from build123d import *

# Parameters (mm, degrees)
CUT_EXTRUDE1_REACH      = 157
SKETCH2_R               = 6
BOSS_EXTRUDE1_DEPTH     = 633
BOSS_EXTRUDE2_DEPTH     = 5
SKETCH6_W               = 63
SKETCH6_H               = 200
BOSS_EXTRUDE3_DEPTH     = 5
BOSS_EXTRUDE4_DEPTH     = 100
CUT_EXTRUDE2_DEPTH      = 128
CUT_EXTRUDE2_DEPTH_BACK = 81


with BuildPart() as part:
    # Sketch1 → Revolve1 (revolve)
    with BuildSketch(Plane(origin=(0, 0, 0), x_dir=(1, 0, 0), z_dir=(0, 1, 0))):
        Polygon((825, 0), (825, 80), (813, 80), (813, 52.102452079), (763.258124913, 43.215384463), (763.258124913, 48.450903374), (746.851230852, 48.450903374), (746.851230852, 33.013608417), (670, 33.013608417), (670, 0), align=None)
    revolve(axis=Axis((657.896171738, 0, 0), (1, 0, 0)))

    # Sketch2 → Cut-Extrude1 (cut, up to next)
    with BuildSketch(Plane(origin=(825, 0, 0), x_dir=(0, 0, -1), z_dir=(1, 0, 0)), mode=Mode.PRIVATE) as cut_extrude1_sk1:
        with Locations((0, 66)):
            Circle(SKETCH2_R)
    cut_extrude1_tool1 = extrude(cut_extrude1_sk1.sketch, amount=-CUT_EXTRUDE1_REACH, mode=Mode.PRIVATE) & part.part
    add(cut_extrude1_tool1.solids().sort_by_distance((825, 66, 0))[0], mode=Mode.SUBTRACT)
    # Sketch2 → Cut-Extrude1 (cut, up to next)
    with BuildSketch(Plane(origin=(825, 0, 0), x_dir=(0, 0, -1), z_dir=(1, 0, 0)), mode=Mode.PRIVATE) as cut_extrude1_sk2:
        with Locations((62.769730075, 20.395121629)):
            Circle(SKETCH2_R)
    cut_extrude1_tool2 = extrude(cut_extrude1_sk2.sketch, amount=-CUT_EXTRUDE1_REACH, mode=Mode.PRIVATE) & part.part
    add(cut_extrude1_tool2.solids().sort_by_distance((825, 20.395122, -62.76973))[0], mode=Mode.SUBTRACT)
    # Sketch2 → Cut-Extrude1 (cut, up to next)
    with BuildSketch(Plane(origin=(825, 0, 0), x_dir=(0, 0, -1), z_dir=(1, 0, 0)), mode=Mode.PRIVATE) as cut_extrude1_sk3:
        with Locations((38.793826651, -53.395121629)):
            Circle(SKETCH2_R)
    cut_extrude1_tool3 = extrude(cut_extrude1_sk3.sketch, amount=-CUT_EXTRUDE1_REACH, mode=Mode.PRIVATE) & part.part
    add(cut_extrude1_tool3.solids().sort_by_distance((825, -53.395122, -38.793827))[0], mode=Mode.SUBTRACT)
    # Sketch2 → Cut-Extrude1 (cut, up to next)
    with BuildSketch(Plane(origin=(825, 0, 0), x_dir=(0, 0, -1), z_dir=(1, 0, 0)), mode=Mode.PRIVATE) as cut_extrude1_sk4:
        with Locations((-38.793826651, -53.395121629)):
            Circle(SKETCH2_R)
    cut_extrude1_tool4 = extrude(cut_extrude1_sk4.sketch, amount=-CUT_EXTRUDE1_REACH, mode=Mode.PRIVATE) & part.part
    add(cut_extrude1_tool4.solids().sort_by_distance((825, -53.395122, 38.793827))[0], mode=Mode.SUBTRACT)
    # Sketch2 → Cut-Extrude1 (cut, up to next)
    with BuildSketch(Plane(origin=(825, 0, 0), x_dir=(0, 0, -1), z_dir=(1, 0, 0)), mode=Mode.PRIVATE) as cut_extrude1_sk5:
        with Locations((-62.769730075, 20.395121629)):
            Circle(SKETCH2_R)
    cut_extrude1_tool5 = extrude(cut_extrude1_sk5.sketch, amount=-CUT_EXTRUDE1_REACH, mode=Mode.PRIVATE) & part.part
    add(cut_extrude1_tool5.solids().sort_by_distance((825, 20.395122, 62.76973))[0], mode=Mode.SUBTRACT)


with BuildPart() as body_2:
    # Sketch4 → Boss-Extrude1 (new body)
    with BuildSketch(Plane(origin=(0, 0, 0), x_dir=(0, 0, -1), z_dir=(1, 0, 0))):
        with BuildLine():
            Line((-185, 107), (-105, 107))
            ThreePointArc((-105, 107), (-97.928932188, 104.071067812), (-95, 97))
            Line((-95, 97), (-95, 37))
            ThreePointArc((-95, 37), (-97.928932188, 29.928932188), (-105, 27))
            Line((-105, 27), (-185, 27))
            ThreePointArc((-185, 27), (-192.071067812, 29.928932188), (-195, 37))
            Line((-195, 37), (-195, 97))
            ThreePointArc((-195, 97), (-192.071067812, 104.071067812), (-185, 107))
        make_face()
    extrude(amount=BOSS_EXTRUDE1_DEPTH)

    # Sketch5 → Boss-Extrude2 (add)
    with BuildSketch(Plane(origin=(633, 0, 0), x_dir=(0, 0, -1), z_dir=(1, 0, 0))):
        Polygon((-245, 127), (-45, 127), (-45, 67), (-115, -3), (-175, -3), (-245, 67), align=None)
    extrude(amount=-BOSS_EXTRUDE2_DEPTH)

    # Sketch6 → Boss-Extrude3 (add)
    with BuildSketch(Plane(origin=(0, 127, 0), x_dir=(1, 0, 0), z_dir=(0, 1, 0))):
        with Locations((601.5, -145)):
            Rectangle(SKETCH6_W, SKETCH6_H)
        with BuildLine():
            Line((595, -58), (605, -58))
            ThreePointArc((605, -58), (612, -65), (605, -72))
            Line((605, -72), (595, -72))
            ThreePointArc((595, -72), (588, -65), (595, -58))
        make_face(mode=Mode.SUBTRACT)
        with BuildLine():
            Line((595, -232), (605, -232))
            ThreePointArc((605, -232), (612, -225), (605, -218))
            Line((605, -218), (595, -218))
            ThreePointArc((595, -218), (588, -225), (595, -232))
        make_face(mode=Mode.SUBTRACT)
    extrude(amount=-BOSS_EXTRUDE3_DEPTH)


with BuildPart() as body_3:
    # Sketch7 → Boss-Extrude4 (new body)
    with BuildSketch(Plane(origin=(633, 0, 0), x_dir=(0, 0, -1), z_dir=(1, 0, 0))):
        with BuildLine():
            Line((-119.363743831, 109.927641091), (17.011140909, 28.484976382))
            ThreePointArc((17.011140909, 28.484976382), (30.118099961, -13.916639292), (-10.667353807, -31.416243525))
            Line((-10.667353807, -31.416243525), (-161.07599492, 19.654858884))
            ThreePointArc((-161.07599492, 19.654858884), (-190.388803142, 87.972757314), (-119.363743831, 109.927641091))
        make_face()
    extrude(amount=BOSS_EXTRUDE4_DEPTH)

    # Sketch8 → Cut-Extrude2 (cut, two sides)
    with BuildSketch(Plane(origin=(0, 0, 0), x_dir=(1, 0, 0), z_dir=(0, 1, 0))) as cut_extrude2_sk:
        Polygon((684.125986069, 52.172184326), (684.125986069, -36.03915177), (633, -87.375021277), (621.083181111, -87.375021277), (621.083181111, 52.172184326), align=None)
        Polygon((762.556990908, -18.927195268), (740.647296939, -18.927195268), (670.961767899, -219.892834515), (762.556990908, -219.892834515), align=None)
    extrude(amount=CUT_EXTRUDE2_DEPTH, mode=Mode.SUBTRACT)
    extrude(cut_extrude2_sk.sketch, amount=-CUT_EXTRUDE2_DEPTH_BACK, mode=Mode.SUBTRACT)


with BuildPart() as body_2_1:
    add(body_2.part)

    # Combine1: union body 3, part
    add(body_3.part)
    add(part.part)

    # Mirror4: body 2 across plane


with BuildPart() as body_2_2:
    add(body_2_1.part)
    add(body_2_1.part.mirror(Plane(origin=(0, 0, 0), x_dir=(0, 0, 1), z_dir=(1, 0, 0))))


solid = body_2_2.part
The listing builds one solid part. Answer for the finished solid, in the listing's coordinates (mm). A direction names the side the tool comes from. Round coordinates to 2 decimals unless told otherwise and drop trailing zeros. Loops run counter-clockwise (first coordinate to the right, second up) from the corner with the lowest first, then second, coordinate; pieces in that order, holes last. Notation, with made-up numbers: M -7,73.5 L 16,73.5 A21 ccw 16,97.5 Z; hole C 5.25,47 d5. An arc over 180 degrees is marked long. Return JSON: item names as keys, results as strings.
Q1. Each of these flat-tipped pins is pushed along its axis until it touches: pin 1 Ø2 at (x, y) = (64.5, 62) entering from -Z; pin 2 Ø10 at (x, z) = (-573, 124) entering from -Y; pin 3 Ø5 at (x, y) = (-315, 102) entering from -Z; pin 4 Ø15.5 at (y, z) = (20.4, 62.77) entering from -X. Where does it stop, or does it pass through?
Results list:
{"pin 1": "stops at z = 95", "pin 2": "stops at y = 27", "pin 3": "stops at z = 95.32", "pin 4": "stops at x = -825"}
Q2. Which of the six approach directions +Z, -Z, +X, -X, +Y, -Y give full straight-line access (tool end or side, diameter ignored) to faces 4 (the face through (-599, 122, 144)), 5 (the face through (706.67, 46.97, 116.91)), 6 (the face through (615, 124, 45)), 7 (the face through (676.964, -32.229, 7.157)), 8 (the face through (-631, 32, 80))?
Results list:
{"face 4": "+Z, -Z", "face 5": "+Z, +Y, -Y", "face 6": "-Z, +X, -X, +Y, -Y", "face 7": "none", "face 8": "-Z, -Y"}
Q3. Find section A-A, the plane x = 188.5. Determine the outline of the cut face in (y, z), plus the area to 3 significant figures.
Results list:
{"outline": "M 27,105 A10 ccw 37,95 L 97,95 A10 ccw 107,105 L 107,185 A10 ccw 97,195 L 37,195 A10 ccw 27,185 Z", "area": "7,910 mm2"}
Q4. Find the intervals of material crossed by line 1 along X through (y, z) = (66, 211); line 2 along X through (y, z) = (-11, -34); line 3 along X through (y, z) = (9, 75.5), in increasing order. Write a range as from..to.
Results list:
{"line 1": "x = -633..-628, 628..633", "line 2": "x = -825..-746.85, 746.85..825", "line 3": "x = -825..-813, -721.03..-644.83, 644.83..721.03, 813..825"}
Q5. The mould has two halves that part along X. Classify faces 1 (the face through (-754.9, -47.3, 10.5)), 2 (the face through (825, 1, -1)), 3 (the face through (-818.92, -78.1, 17.34)): released by +X, released by -X, zero draft, split by the parting line, or undercut.
Results list:
{"face 1": "undercut", "face 2": "released by +X", "face 3": "zero draft"}
